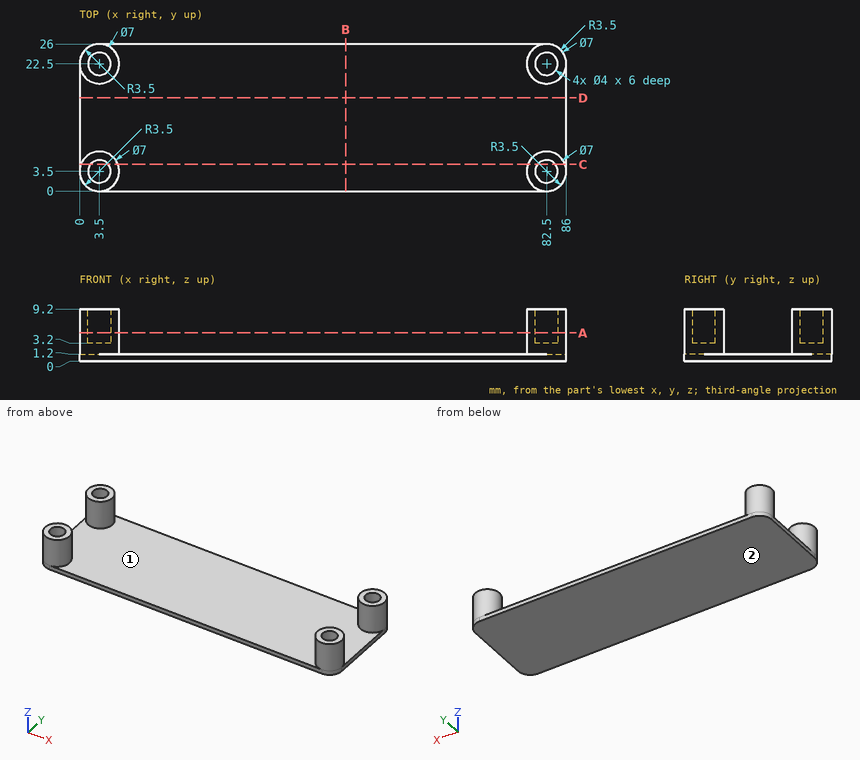
Job drawing, mm, ordinate dimensions from the low corner. One solid piece. Round coordinates to 2 decimals unless told otherwise and drop trailing zeros. Loops run counter-clockwise (first coordinate to the right, second up) from the corner with the lowest first, then second, coordinate; pieces in that order, holes last.
(1) Two-plate mould, pull along X, no slides. Class the marked faces 1 and 2: +X half, -X half, draft (parallel to the pull), parting line (faces both ways), or undercut.
(2) Cut at D-D (y = 16.5). Give the cut face in (x, z).
(3) Wall check: line 1 along Y through (x, z) = (3.5, 5.4); line 2 along X through (y, z) = (23, 6); line 3 along Z through (x, y) = (78, 23). Give the ranges that are in metal, low to high.
(4) Cut at B-B (x = 47). Give the cut face in (y, z), plus the area to 3 significant figures.
(5) Cut at C-C (y = 4.75). Give the cut face in (x, z), plus the area to 3 significant figures.
(6) Cut at A-A (z = 5). Give the cut face in (x, y).
(7) Drop flat-ended pins along their axis: pin 1 (3 mm diameter, centred on x = 42, y = 3.5, fed in from +Z); pin 2 (4.5 mm diameter, centred on x = 82.5, y = 22.5, fed in from +Z); pin 3 (1.5 mm diameter, centred on y = 9.5, z = 2, fed in from -X); pin 4 (1.2 mm diameter, centred on x = 4, y = 22, fed in from +Z). Give the stop position or say it passes through.
Findings below:
1. face 1: undercut
1. face 2: draft
2. outline: (0, 0) - (86, 0) - (86, 1.2) - (0, 1.2) - close
3. line 1: y = 0 to 1.5, 5.5 to 7, 19 to 20.5, 24.5 to 26
3. line 2: x = 0.04 to 1.56, 5.44 to 6.96, 79.04 to 80.56, 84.44 to 85.96
3. line 3: z = 0 to 1.2
4. outline: (0, 0) - (26, 0) - (26, 1.2) - (0, 1.2) - close
4. area: 31.2 mm2
5. outline: (0, 0) - (86, 0) - (86, 1.2) - (85.77, 1.2) - (85.77, 9.2) - (84.06, 9.2) - (84.06, 3.2) - (80.94, 3.2) - (80.94, 9.2) - (79.23, 9.2) - (79.23, 1.2) - (6.77, 1.2) - (6.77, 9.2) - (5.06, 9.2) - (5.06, 3.2) - (1.94, 3.2) - (1.94, 9.2) - (0.23, 9.2) - (0.23, 1.2) - (0, 1.2) - close
5. area: 170 mm2
6. outline: circle Ø7 at (3.5, 3.5); circle Ø7 at (3.5, 22.5); circle Ø7 at (82.5, 3.5); circle Ø7 at (82.5, 22.5); hole circle Ø4 at (3.5, 3.5); hole circle Ø4 at (3.5, 22.5); hole circle Ø4 at (82.5, 3.5); hole circle Ø4 at (82.5, 22.5)
7. pin 1: stops at z = 1.2
7. pin 2: stops at z = 9.2
7. pin 3: passes through
7. pin 4: stops at z = 3.2
